Autodesk Inventor part; units mm, degrees
ref_plane "YZ Plane" through (0, 0, 0) normal (1, 0, 0) x (0, 1, 0)
ref_plane "XZ Plane" through (0, 0, 0) normal (0, 1, 0) x (-1, 0, 0)
ref_plane "XY Plane" through (0, 0, 0) normal (0, 0, 1) x (1, 0, 0)
sketch "Sketch1" plane through (0, 0, 0) normal (0, 1, 0) x (-1, 0, 0)
  line L0 (-2.2837, -0.9982) -> (0.008, -0.7055) construction
  line L1 (2.6844, -8.3272) -> (2.6844, -12.3272) construction
  line L2 (64.2192, 40.0403) -> (72.5206, 41.3734) construction
  line L3 (64.2192, 39.2192) -> (64.2192, 44.778) construction
  line L4 (-8.9125, -2.5) -> (-8.9125, -6.85) construction
  line L5 (-14.9605, -0.9982) -> (-2.2837, -0.9982) construction
  line L6 (55.95, 41.2553) -> (64.2192, 40.0403) construction
  circle A0 centre (-8.9125, -6.85) radius 4.35
  line L7 (-14.724, -20.8143) -> (-17.8001, -0.7055) construction
  line L8 (-3.0681, -20.8143) -> (0.008, -0.7055) construction
  line L9 (-11.8961, -14.832) -> (-8.8961, -13.1) construction
  line L10 (-8.8961, -13.1) -> (-5.8961, -14.832) construction
  line L11 (-3.0681, -20.8143) -> (-14.724, -20.8143)
  circle A1 centre (-8.8961, -16.5641) radius 1.9
  line L12 (64.2192, 39.2192) -> (64.2192, 43.7357)
  line L13 (-14.9605, -0.9982) -> (-17.8001, -0.7055) construction
  line L14 (-8.8961, -20.8143) -> (-3.0681, -20.8143) construction
  line L15 (-14.724, -20.8143) -> (-3.0681, -20.8143) construction
  line L16 (-8.8258, -6.8795) -> (-8.8093, -6.8795) construction
  line L17 (-5.8961, -14.832) -> (-5.3727, -20.8143) construction
  line L18 (-11.8961, -14.832) -> (-12.4194, -20.8143) construction
  line L19 (-14.2025, 0) -> (-14.2025, -2.5) construction
  line L20 (-14.2025, -2.5) -> (-3.6225, -2.5) construction
  line L21 (-8.9125, -2.5) -> (-8.9125, 0.8916) construction
  line L22 (-3.6225, -20.8143) -> (-14.2025, -20.8143) construction
  line L23 (-3.6225, -20.8143) -> (-14.2025, -20.8143)
  line L24 (-8.9125, -6.85) -> (-13.2625, -6.85) construction
  line L25 (-13.2625, -6.85) -> (-14.2025, -6.85) construction
  line L26 (-3.0681, -20.8143) -> (-3.0681, 0)
  line L27 (-14.724, -20.8143) -> (-14.724, 0) construction
  line L28 (-14.724, 0) -> (-14.2025, 0) construction
  line L29 (-14.724, -20.8143) -> (-14.724, 0)
  line L30 (-14.2025, 0) -> (-14.724, 0)
  line L31 (-3.0681, 0) -> (-3.0681, 4)
  line L32 (-3.0681, 4) -> (-14.724, 4)
  line L33 (-14.724, 0) -> (-14.724, 4)
  point P0 (-0.8016, -0.9982)
  point P1 (-16.9905, -0.9982)
  point P2 (-5.8961, -16.5641)
  point P3 (-8.8961, -16.5641)
  point P4 (-11.8961, -20.8143)
  point P5 (-5.8961, -20.8143)
  dimension "d27" = 3.8
  dimension "d28" = 4
  dimension "d29" = 0.0164
  dimension "d31" = 2.5
  dimension "d36" = 4
extrude "Extrusion1" add sketch "Sketch1" along normal blind 2
sketch "Sketch5" plane through (3.0681, 0, 4) normal (0, 0, 1) x (1, 0, 0)
  line L0 (5.6876, -20.2886) -> (8.131, -18.0087) construction
  line L1 (5.8983, -14.0653) -> (5.9147, -14.0653) construction
  line L2 (0, -28) -> (-3.0761, -7.8912) construction
  circle A0 centre (5.8115, -14.0357) radius 4.35
  line L3 (11.6559, -28) -> (14.732, -7.8912) construction
  line L4 (5.8115, -9.6857) -> (5.8115, -14.0357) construction
  line L5 (-22.6444, -7.0488) -> (-20.3527, -6.7561) construction
  circle A1 centre (5.828, -23.7498) radius 1.9
  line L6 (2.828, -22.0178) -> (2.3046, -28) construction
  line L7 (11.6559, -28) -> (0, -28) construction
  line L8 (0, -28) -> (11.6559, -28) construction
  line L9 (5.828, -28) -> (11.6559, -28) construction
  line L10 (8.131, -18.0087) -> (9.3514, -28) construction
  line L11 (2.828, -22.0178) -> (5.6876, -20.2886) construction
  line L12 (-35.3212, -7.0488) -> (-22.6444, -7.0488) construction
  line L13 (-35.3212, -7.0488) -> (-38.1608, -6.7561) construction
  line L14 (0.5215, -7.1857) -> (0.5215, -9.6857) construction
  line L15 (0.5215, -9.6857) -> (11.1015, -9.6857) construction
  line L16 (5.8115, -9.6857) -> (5.8115, -6.2941) construction
  line L17 (11.1015, -28) -> (0.5215, -28) construction
  line L18 (11.1015, -28) -> (0.5215, -28) construction
  line L19 (5.8115, -14.0357) -> (1.4615, -14.0357) construction
  line L20 (1.4615, -14.0357) -> (0.5215, -14.0357) construction
  line L21 (11.6559, -28) -> (11.6559, -7.1857) construction
  line L22 (0, -28) -> (0, -7.1857) construction
  line L23 (-35.0847, -6.0506) -> (-34.5632, -6.0506) construction
  line L24 (0, -28) -> (0, -7.1857) construction
  line L25 (-34.5632, -6.0506) -> (-35.0847, -6.0506) construction
  line L26 (-23.4288, -6.0506) -> (-23.4288, -2.0506) construction
  line L27 (-23.4288, -2.0506) -> (-35.0847, -2.0506) construction
  line L28 (-35.0847, -6.0506) -> (-35.0847, -2.0506) construction
  line L29 (0, 0) -> (11.6559, 0)
  line L30 (11.6559, 0) -> (11.6559, 2)
  line L31 (0, 2) -> (11.6559, 2)
  line L32 (0, 0) -> (0, 2)
  line L33 (0, 2) -> (11.6559, 2)
  line L34 (11.6559, 2) -> (11.6559, -28)
  line L35 (11.6559, -28) -> (0, -28)
  line L36 (0, -28) -> (0, 2)
  line L37 (5.828, -28) -> (5.828, -33.9662)
  line L38 (5.828, -28) -> (5.7489, -34.6939)
  point P0 (-4.0686, -7.3836)
  point P1 (8.828, -23.7498)
  point P2 (2.828, -28)
  point P3 (8.828, -28)
  point P4 (-37.3512, -7.0488)
  dimension "d38" = 3.8
  dimension "d40" = 0.0164
  dimension "d41" = 2.5
  dimension "d42" = 4
  dimension "d43" = 30
extrude "Extrusion5" add sketch "Sketch5" along normal blind 2
sketch "Sketch6" plane through (3.0681, 0, 4) normal (0, 0, -1) x (-1, 0, 0)
  line L0 (0, 0) -> (-11.6559, 0)
  line L1 (-11.6559, -28) -> (-11.6559, 0)
  line L2 (0, -28) -> (-11.6559, -28)
  line L3 (0, 0) -> (0, -28)
  circle A0 centre (-5.828, -23.7498) radius 1.9
  circle A1 centre (-5.8115, -14.0357) radius 4.35
  circle A2 centre (-5.8115, -14.0357) radius 4.35
  circle A3 centre (-5.8115, -14.0357) radius 5.8444
  line L4 (-11.6559, -28) -> (-11.6559, 0)
  point P0 (3.0681, 0)
extrude "Extrusion6" add sketch "Sketch6" along normal blind 3.5 contours A3 L3 | L3 A3
chamfer "Chamfer1" distance 0.5 distance2 3.5 1 edges at (14.724, -14.0357, 0.5) measured on face at (3.6321, -14.849, 0.5)
sketch "Sketch8" plane through (0, 0, 0) normal (0, -1, 0) x (1, 0, 0)
  circle A0 centre (8.9125, -6.85) radius 4.35
  circle A1 centre (8.8961, -16.5641) radius 1.9
  line L0 (14.724, -20.8143) -> (3.0681, -20.8143)
  line L1 (14.724, 4) -> (14.724, -20.8143)
  line L2 (3.0681, 4) -> (14.724, 4)
  line L3 (3.0681, -20.8143) -> (3.0681, 4)
  arc A2 (3.0681, -6.85) -> (14.724, -7.4691) centre (8.9125, -6.85) ccw
  line L4 (48.394, -18.4641) -> (53.1571, -15.7141)
  line L5 (51.5694, -18.4641) -> (49.9817, -21.2141)
  line L6 (49.9817, -21.2141) -> (46.8063, -21.2141)
  line L7 (46.8063, -21.2141) -> (45.2186, -18.4641)
  line L8 (45.2186, -18.4641) -> (46.8063, -15.7141)
  line L9 (46.8063, -15.7141) -> (49.9817, -15.7141)
  line L10 (49.9817, -15.7141) -> (51.5694, -18.4641)
  line L11 (8.8961, -16.5641) -> (13.6592, -13.8141)
  line L12 (12.0715, -16.5641) -> (10.4838, -19.3141)
  line L13 (10.4838, -19.3141) -> (7.3083, -19.3141)
  line L14 (7.3083, -19.3141) -> (5.7206, -16.5641)
  line L15 (5.7206, -16.5641) -> (7.3083, -13.8141)
  line L16 (7.3083, -13.8141) -> (10.4838, -13.8141)
  line L17 (10.4838, -13.8141) -> (12.0715, -16.5641)
  point P0 (0, 0)
  point P1 (50.7756, -17.0891)
  point P2 (11.2776, -15.1891)
  dimension "d53" = 5.5
  dimension "d54" = 5.5
extrude "Extrusion7" add sketch "Sketch8" along normal blind 3.5 contours A2 L3 L2 L1
properties part number "Now as three El L"
Part model, mm, in its own coordinate system. A direction names the side the tool comes from. Coordinates: 2 decimals unless noted, no trailing zeros. Loops run counter-clockwise (first coordinate to the right, second up) from the corner with the lowest first, then second, coordinate; pieces in that order, holes last. Notation, with made-up numbers: (-13.5, 87) - (-4.5, 87) arc R21 cw to (-4.5, 97) - close; hole circle Ø7 at (37, 71). An arc over 180 degrees is marked (long way). Write item = value, one per line. Start each with the question number.
Item 1: Wall check: L1, parallel to X at y = -1.15, z = -6.85; L2, parallel to Y at x = 5.5, z = 1; L3, parallel to Z at x = 10.5, y = 0.5. Give the ranges that are in metal, low to high. Write a range as from..to.
Item 2: Cut at B-B, the plane y = -21.25. Give the cut face in (x, z).
Item 3: Cut at C-C, the plane x = 6.5. State how many separate pieces and enclosed holes the cut face has, and give its area (3 significant figures).
Item 4: Cut at A-A, the plane z = -4.75. Give the cut face in (x, y), and give its area (3 significant figures).
Item 5: Cut at D-D, the plane z = -1.5. Give the cut face in (x, y).
Item 6: Mould opens along X. For faces 5 (the cylindrical face through (8.02, 0.99, -14.88)), 6 (the conical face through (10.07, -8.68, 1.5)), 7 (the flat face through (9, 1, -20.814)), 8 (the cylindrical face through (8.649, -25.634, 4.986)) say: released by +X, released by -X, zero draft, split by the parting line, or undercut.
Item 7: Flat gauge pins, fed straight in: pin 1 Ø4 at (y, z) = (-16.5, -0.5) entering from +X; pin 2 Ø6 at (x, z) = (8.9, -16.56) entering from -Y; pin 3 Ø3.5 at (x, y) = (10, -19) entering from -Z. Where does each tip first touch, or does it go through?
Item 8: 3-axis set-ups, long thin cutter, end or side, ignore diameter. For faces 1 (the flat face through (14.724, -3, -1)), 2 (the flat face through (7.7, -18.4, 0.5)), 3 (the cylindrical face through (8.73, -1.73, -12.69)), 4 (the flat face through (9, -3.5, -2)): which of +Z, -Z, +X, -X, +Y, -Y reach the whole face in a straight line?
The answers:
q1.L1 = 3.07..4.56, 13.26..14.72
q1.L2 = -18.27..-16.77, -11.3..-9.8, -3.5..2
q1.L3 = -20.81..-17.58, -15.55..-10.9, -2.8..6
q2.outline = (3.07, 4) - (14.72, 4) - (14.72, 6) - (3.07, 6) - close
q3.separate_pieces = 3
q3.enclosed_holes = 0
q3.area = 122 mm2
q4.outline = (3.07, -3.5) - (5.1, -3.5) - (5.1, 2) - (3.07, 2) - close; (12.72, -3.5) - (14.72, -3.5) - (14.72, 2) - (12.72, 2) - close
q4.area = 22.2 mm2
q5.outline = (3.07, -3.5) - (14.72, -3.5) - (14.72, 2) - (3.07, 2) - close
q6.face_5 = undercut
q6.face_6 = split by the parting line
q6.face_7 = zero draft
q6.face_8 = undercut
q7.pin_1 = 14.18
q7.pin_2 = 0
q7.pin_3 = 0.5
q8.face_1 = +Z, -Z, +X, +Y, -Y
q8.face_2 = -Z, +X, -X, -Y
q8.face_3 = -Z, -Y
q8.face_4 = -Z, +X, -X
